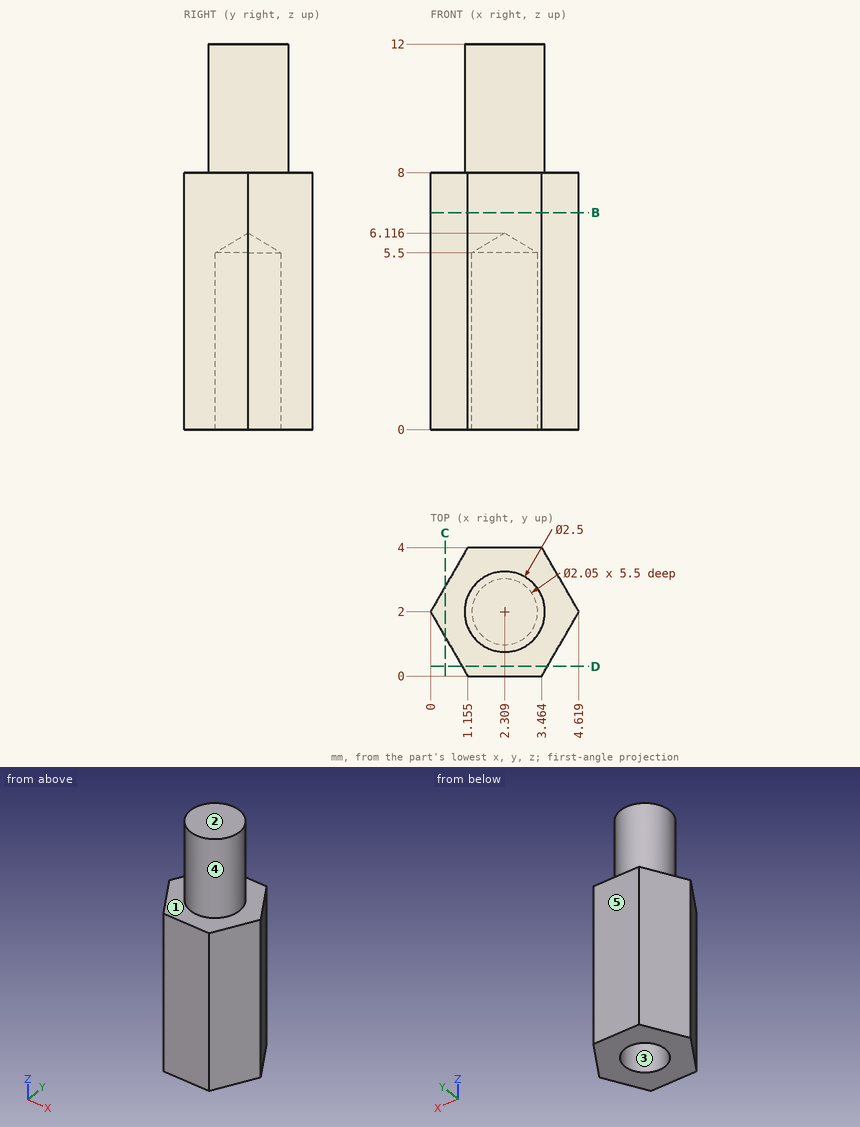
For this review, use the dimensioned drawing (mm, ordinates from the lowest corner) and the shaded views. A direction names the side the tool comes from. Round coordinates to 2 decimals unless told otherwise and drop trailing zeros. Order: outer loops, then holes, each group sorted by start corner. A loop starts at its lowest first (then second) coordinate and runs counter-clockwise, first axis right, second up. Notation, with made-up numbers: (70, -26.5) - (91, -26.5) arc R10 cw to (91, -16.5) - close; hole circle Ø9 at (-26, 61). An arc over 180 degrees is marked (long way). Use one line per item in the form item = value.
Q1. Add section D-D on y = 0.3. Give the boundary of the cut face in (x, z).
Response values:
outline = (0.98, 0) - (3.64, 0) - (3.64, 8) - (0.98, 8) - close
Q2. Add section B-B on z = 6.75. Give the boundary of the cut face in (x, y) (1 decimal).
Response values:
outline = (0, 2) - (1.2, 0) - (3.5, 0) - (4.6, 2) - (3.5, 4) - (1.2, 4) - close
Q3. Add section C-C on x = 0.45. Give the boundary of the cut face in (y, z).
Response values:
outline = (1.22, 0) - (2.78, 0) - (2.78, 8) - (1.22, 8) - close
Q4. Clearance check with flat-ended pins moving along their axes: P1, Ø1.5, axis at y = 1.5, z = 9.5, coming from the -X side; P2, Ø1, axis at y = 3, z = 6, coming from the +X side. State where each tip first meets the part, or that it passes through.
Response values:
P1 = 1.06
P2 = 4.33
Q5. Tool access review of the marked faces 1 and 2: name each direction out of +Z, -Z, +X, -X, +Y, -Y from which nothing blocks a thin tool from reaching the whole face with its end or side.
Response values:
face_1 = +Z
face_2 = +Z, +X, -X, +Y, -Y
Q6. To check wall thickness, follow line 1 (Z direction, x = 1.3, y = 3.55); line 2 (Y direction, x = 1.95, z = 3.5); line 3 (Y direction, x = 1.55, z = 3.5). State the ranges of each line that lie inside material, in increasing order.
Response values:
line_1 = 0 to 8
line_2 = 0 to 1.04, 2.96 to 4
line_3 = 0 to 1.31, 2.69 to 4
Q7. Mouldability with a two-part tool opening along Y and no side actions: class the marked faces 3, 4 and 5 as pulls with the +Y half, pulls with the -Y half, needs draft (parallel to the pull), parting line crosses it, or undercut.
Response values:
face_3 = undercut
face_4 = parting line crosses it
face_5 = pulls with the +Y half
